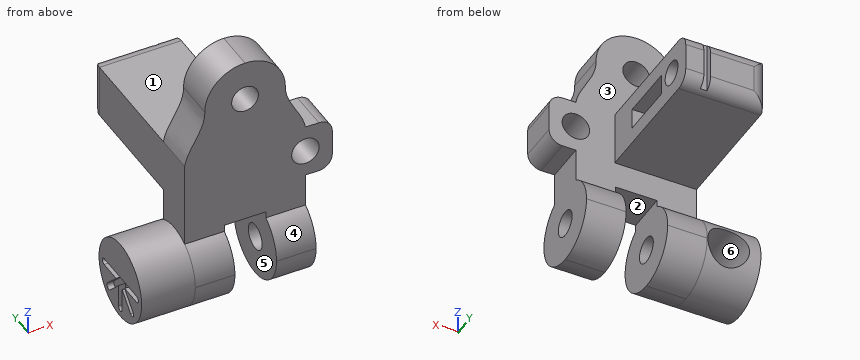
from build123d import *

# Parameters (mm, degrees)
SKETCH1_W           = 9
SKETCH1_H           = 9
BOSS_EXTRUDE1_DEPTH = 3
SKETCH2_W           = 2.95
SKETCH2_H           = 6
BOSS_EXTRUDE2_DEPTH = 6.1
FILLET1_R           = 3
SKETCH3_R           = 0.975
CUT_EXTRUDE1_DEPTH  = 11.1
CUT_EXTRUDE3_DEPTH  = 21.1
BOSS_EXTRUDE3_START = 4
SKETCH5_R           = 3
BOSS_EXTRUDE3_DEPTH = 4
SKETCH8_R           = 1.55
CUT_EXTRUDE4_DEPTH  = 5
CUT_EXTRUDE5_DEPTH  = 0.5
SKETCH10_W          = 9
SKETCH10_H          = 3
BOSS_EXTRUDE4_DEPTH = 4
SKETCH11_R          = 1
CUT_EXTRUDE6_DEPTH  = 4
CUT_EXTRUDE7_DEPTH  = 4
SKETCH13_W          = 6.1
SKETCH13_H          = 4
BOSS_EXTRUDE7_DEPTH = 7.5
SKETCH16_W          = 1.55
SKETCH16_H          = 4.1
CUT_EXTRUDE9_DEPTH  = 3.2
SKETCH17_W          = 4
SKETCH17_H          = 3
BOSS_EXTRUDE8_DEPTH = 2
SKETCH19_R          = 1.025
CUT_EXTRUDE10_DEPTH = 4
FILLET2_R           = 1
SKETCH21_W          = 6.1
SKETCH21_H          = 4
BOSS_EXTRUDE9_DEPTH = 2.5
SKETCH23_R          = 0.9
CUT_EXTRUDE11_DEPTH = 4
FILLET3_R           = 1
CUT_EXTRUDE12_DEPTH = 0.5


with BuildPart() as part:
    # Sketch1 → Boss-Extrude1 (new body)
    with BuildSketch(Plane(origin=(0, 0, 0), x_dir=(1, 0, 0), z_dir=(0, 1, 0))):
        with Locations((4.5, 4.5)):
            Rectangle(SKETCH1_W, SKETCH1_H)
    extrude(amount=BOSS_EXTRUDE1_DEPTH)

    # Sketch2 → Boss-Extrude2 (add)
    with BuildSketch(Plane(origin=(0, 0, -9), x_dir=(-1, 0, 0), z_dir=(0, 0, -1))):
        with Locations((-7.525, 1.5)):
            Rectangle(SKETCH2_W, SKETCH2_H)
        with Locations((-1.475, 1.5)):
            Rectangle(SKETCH2_W, SKETCH2_H)
    extrude(amount=BOSS_EXTRUDE2_DEPTH)

    # Fillet1
    fillet1_edges = [part.edges().sort_by_distance(p)[0] for p in [
        (1.475, 4.5, -15.1),
        (1.475, -1.5, -15.1),
        (7.525, -1.5, -15.1),
        (7.525, 4.5, -15.1),
    ]]
    fillet(fillet1_edges, radius=FILLET1_R - 0.0001)  # a hair under: the kernel refuses the full size

    # Sketch3 → Cut-Extrude1 (cut)
    with BuildSketch(Plane(origin=(9, 0, 0), x_dir=(0, 0, -1), z_dir=(1, 0, 0))):
        with Locations((12.1, 1.5)):
            Circle(SKETCH3_R)
    extrude(amount=-CUT_EXTRUDE1_DEPTH, mode=Mode.SUBTRACT)

    # Sketch6 → Cut-Extrude3 (cut)
    with BuildSketch(Plane.ZY):
        with BuildLine():
            Line((-12.1, 4.5), (-9, 4.5))
            Line((-9, 4.5), (-9, 3))
            Line((-9, 3), (-9.501923789, 3))
            ThreePointArc((-9.501923789, 3), (-10.6, 4.098076211), (-12.1, 4.5))
        make_face()
        with BuildLine():
            Line((-12.1, -1.5), (-9, -1.5))
            Line((-9, -1.5), (-9, 0))
            Line((-9, 0), (-9.501923789, 0))
            ThreePointArc((-9.501923789, 0), (-10.6, -1.098076211), (-12.1, -1.5))
        make_face()
    extrude(amount=-CUT_EXTRUDE3_DEPTH, mode=Mode.SUBTRACT)

    # Sketch5 → Boss-Extrude3 (add)
    with BuildSketch(Plane.ZY.offset(BOSS_EXTRUDE3_START)):
        with Locations((-12.1, 1.5)):
            Circle(SKETCH5_R)
    extrude(amount=-BOSS_EXTRUDE3_DEPTH)

    # Sketch8 → Cut-Extrude4 (cut)
    with BuildSketch(Plane(origin=(0, 4.5, 0), x_dir=(-1, 0, 0), z_dir=(0, -1, 0))):
        with Locations(Location((1.6, 12.1, 0), (0, 0, 270))):
            Circle(SKETCH8_R)
    extrude(amount=CUT_EXTRUDE4_DEPTH, mode=Mode.SUBTRACT)

    # Sketch9 → Cut-Extrude5 (cut)
    with BuildSketch(Plane.ZY.offset(4)):
        with BuildLine():
            Line((-11.85, 1.5), (-11.85, -0.8))
            ThreePointArc((-11.85, -0.8), (-12.1, -1.05), (-12.35, -0.8))
            Line((-12.35, -0.8), (-12.35, 0.896446609))
            Line((-12.35, 0.896446609), (-13.549568901, -0.303122292))
            ThreePointArc((-13.549568901, -0.303122292), (-13.903122292, -0.303122292), (-13.903122292, 0.050431099))
            Line((-13.903122292, 0.050431099), (-12.703553391, 1.25))
            Line((-12.703553391, 1.25), (-14.4, 1.25))
            ThreePointArc((-14.4, 1.25), (-14.65, 1.5), (-14.4, 1.75))
            Line((-14.4, 1.75), (-12.703553391, 1.75))
            Line((-12.703553391, 1.75), (-13.903122292, 2.949568901))
            ThreePointArc((-13.903122292, 2.949568901), (-13.903122292, 3.303122292), (-13.549568901, 3.303122292))
            Line((-13.549568901, 3.303122292), (-12.35, 2.103553391))
            Line((-12.35, 2.103553391), (-12.35, 3.8))
            ThreePointArc((-12.35, 3.8), (-12.1, 4.05), (-11.85, 3.8))
            Line((-11.85, 3.8), (-11.85, 1.5))
        make_face()
    extrude(amount=-CUT_EXTRUDE5_DEPTH, mode=Mode.SUBTRACT)

    # Sketch10 → Boss-Extrude4 (add)
    with BuildSketch(Plane.XY):
        with Locations((4.5, 1.5)):
            Rectangle(SKETCH10_W, SKETCH10_H)
    extrude(amount=BOSS_EXTRUDE4_DEPTH)

    # Sketch11 → Cut-Extrude6 (cut)
    with BuildSketch(Plane(origin=(0, 3, 0), x_dir=(1, 0, 0), z_dir=(0, 1, 0))):
        with Locations(Location((4.5, -1, 0), (0, 0, 270))):
            Circle(SKETCH11_R)
    extrude(amount=-CUT_EXTRUDE6_DEPTH, mode=Mode.SUBTRACT)

    # Sketch12 → Cut-Extrude7 (cut)
    with BuildSketch(Plane(origin=(0, 3, 0), x_dir=(1, 0, 0), z_dir=(0, 1, 0))):
        with BuildLine():
            add(Edge.make_bspline(
                [(1.5, -1), (1.53988428, 0.555027292), (0.235256098, 1.545486909), (0, 3)],
                knots=[0, 0, 0, 0, 1, 1, 1, 1], degree=3))
            Line((0, 3), (0, -4))
            Line((0, -4), (4.5, -4))
            ThreePointArc((4.5, -4), (2.378679656, -3.121320344), (1.5, -1))
        make_face()
        with BuildLine():
            ThreePointArc((7.5, -1), (6.621320344, -3.121320344), (4.5, -4))
            Line((4.5, -4), (9, -4))
            Line((9, -4), (9, 3))
            add(Edge.make_bspline(
                [(7.5, -1), (7.46011572, 0.555027292), (8.764743902, 1.545486909), (9, 3)],
                knots=[0, 0, 0, 0, 1, 1, 1, 1], degree=3))
        make_face()
    extrude(amount=-CUT_EXTRUDE7_DEPTH, mode=Mode.SUBTRACT)

    # Sketch13 → Boss-Extrude7 (add)
    with BuildSketch(Plane(origin=(0, 3, 0), x_dir=(1, 0, 0), z_dir=(0, 1, 0))):
        with Locations((3.05, 5)):
            Rectangle(SKETCH13_W, SKETCH13_H)
    extrude(amount=BOSS_EXTRUDE7_DEPTH)

    # Sketch16 → Cut-Extrude9 (cut)
    with BuildSketch(Plane(origin=(6.1, 0, 0), x_dir=(0, 0, -1), z_dir=(1, 0, 0))):
        with Locations((5, 7.5)):
            Rectangle(SKETCH16_W, SKETCH16_H)
    extrude(amount=-CUT_EXTRUDE9_DEPTH, mode=Mode.SUBTRACT)

    # Sketch17 → Boss-Extrude8 (add)
    with BuildSketch(Plane(origin=(9, 0, 0), x_dir=(0, 0, -1), z_dir=(1, 0, 0))):
        with Locations((5, 1.5)):
            Rectangle(SKETCH17_W, SKETCH17_H)
    extrude(amount=BOSS_EXTRUDE8_DEPTH)

    # Sketch19 → Cut-Extrude10 (cut)
    with BuildSketch(Plane(origin=(0, 3, 0), x_dir=(1, 0, 0), z_dir=(0, 1, 0))):
        with Locations(Location((9, 5, 0), (0, 0, 270))):
            Circle(SKETCH19_R)
    extrude(amount=-CUT_EXTRUDE10_DEPTH, mode=Mode.SUBTRACT)

    # Fillet2
    fillet2_edges = [part.edges().sort_by_distance(p)[0] for p in [
        (11, 1.5, -3),
        (11, 1.5, -7),
    ]]
    fillet(fillet2_edges, radius=FILLET2_R)

    # Sketch21 → Boss-Extrude9 (add)
    with BuildSketch(Plane(origin=(0, 10.5, 0), x_dir=(1, 0, 0), z_dir=(0, 1, 0))):
        with Locations((3.05, 5)):
            Rectangle(SKETCH21_W, SKETCH21_H)
    extrude(amount=BOSS_EXTRUDE9_DEPTH)

    # Sketch23 → Cut-Extrude11 (cut)
    with BuildSketch(Plane(origin=(6.1, 0, 0), x_dir=(0, 0, -1), z_dir=(1, 0, 0))):
        with Locations((5, 11)):
            Circle(SKETCH23_R)
    extrude(amount=-CUT_EXTRUDE11_DEPTH, mode=Mode.SUBTRACT)

    # Fillet3
    fillet3_edges = [part.edges().sort_by_distance(p)[0] for p in [
        (3.05, 13, -7),
        (0, 13, -5),
        (3.05, 13, -3),
    ]]
    fillet(fillet3_edges, radius=FILLET3_R)

    # Sketch24 → Cut-Extrude12 (cut)
    with BuildSketch(Plane(origin=(0, 13, 0), x_dir=(1, 0, 0), z_dir=(0, 1, 0))):
        with BuildLine():
            Line((4.25, 3), (4.25, 7))
            ThreePointArc((4.25, 7), (4.5, 7.25), (4.75, 7))
            Line((4.75, 7), (4.75, 3))
            ThreePointArc((4.75, 3), (4.5, 2.75), (4.25, 3))
        make_face()
    extrude(amount=-CUT_EXTRUDE12_DEPTH, mode=Mode.SUBTRACT)


solid = part.part
Geometry check sheet. Reference: the model listing, model coordinates, mm. Face numbers are marked on the shaded views. A direction names the side the tool comes from. Round coordinates to 2 decimals unless told otherwise and drop trailing zeros. Loops run counter-clockwise (first coordinate to the right, second up) from the corner with the lowest first, then second, coordinate; pieces in that order, holes last. Notation, with made-up numbers: (23, -29) - (64, -29) arc R25 ccw to (64, -4) - close; hole circle Ø2 at (24.5, -3.5). An arc over 180 degrees is marked (long way). Answer as CSV lines item,"result".
(1) Cross-section at C-C, the plane y = 11. Enter the section's corners in (x, z).
Output values:
outline,"(0, -7) - (6.1, -7) - (6.1, -5.9) - (2.1, -5.9) - (2.1, -4.1) - (6.1, -4.1) - (6.1, -3) - (0, -3) - close"
(2) Cross-section at B-B, the plane x = 9.5. Enter the section's corners in (y, z).
Output values:
outline,"(0, -7) - (3, -7) - (3, -5.89) - (0, -5.89) - close; (0, -4.11) - (3, -4.11) - (3, -3) - (0, -3) - close"
(3) Material ranges on line 1 along X through (y, z) = (-1, -10.5); line 2 along X through (y, z) = (0.65, -5) (3 decimals); line 3 along X through (y, z) = (12, -4.75), recorded low to high.
Output values:
line 1,"x = -4 to 2.95, 6.05 to 9"
line 2,"x = 0 to 7.975, 10.025 to 11"
line 3,"x = 0 to 6.1"
(4) Cross-section at A-A, the plane z = -5. Enter the section's corners in (x, y) (3 decimals), and give its area (3 significant figures).
Output values:
outline,"(0, 0) - (7.975, 0) - (7.975, 3) - (6.1, 3) - (6.1, 5.45) - (2.9, 5.45) - (2.9, 9.55) - (6.1, 9.55) - (6.1, 10.1) - (2.1, 10.1) - (2.1, 11.9) - (6.1, 11.9) - (6.1, 13) - (4.75, 13) - (4.75, 12.5) - (4.25, 12.5) - (4.25, 13) - (1, 13) arc R1 ccw to (0, 12) - close; (10.025, 0) - (11, 0) - (11, 3) - (10.025, 3) - close"
area,"67.1 mm²"
(5) Set-up check for the marked faces 1, 2 and 3: record each of +Z, -Z, +X, -X, +Y, -Y from which the full face is reachable in a straight line by a thin tool's end or side.
Output values:
face 1,"+Z, +X, -X, +Y"
face 2,"-Z, +Y, -Y"
face 3,"+X, +Y"
(6) Release check for a two-part mould opening along Z. For the marked faces 4, 5 and 6 record: released by +Z, released by -Z, zero draft, split by the parting line, or undercut.
Output values:
face 4,"released by +Z"
face 5,"zero draft"
face 6,"undercut"
(7) Depth check by flat-ended pin: pin 1 Ø0.6 at (y, z) = (12.5, -4.5) entering from -X; pin 2 Ø1.2 at (y, z) = (6, -5) entering from +X; pin 3 Ø1.2 at (y, z) = (1.5, -12.1) entering from +X. Enter the tip coordinate at first touch or a pass-through.
Output values:
pin 1,"stops at x = 0.02"
pin 2,"stops at x = 6.1"
pin 3,"stops at x = 0"
